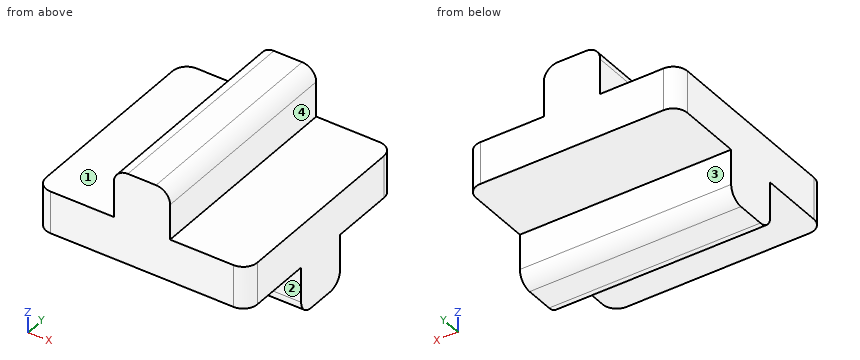
from build123d import *

# Parameters (mm, degrees)
SKETCH_1_W      = 30
SKETCH_1_H      = 30
EXTRUDE_1_DEPTH = 6
SKETCH_2_W      = 30
SKETCH_2_H      = 8
EXTRUDE_2_DEPTH = 7
FILLET_1_R      = 2
FILLET_2_R      = 2
SKETCH_3_W      = 8
SKETCH_3_H      = 30
EXTRUDE_3_DEPTH = 7
FILLET_3_R      = 2


with BuildPart() as part:
    # 스케치1 → 보스-돌출1 (new body)
    with BuildSketch(Plane.XY):
        Rectangle(SKETCH_1_W, SKETCH_1_H)
    extrude(amount=EXTRUDE_1_DEPTH)

    # 스케치2 → 보스-돌출2 (add)
    with BuildSketch(Plane(origin=(0, 0, 0), x_dir=(-1, 0, 0), z_dir=(0, 0, -1))):
        Rectangle(SKETCH_2_W, SKETCH_2_H)
    extrude(amount=EXTRUDE_2_DEPTH)

    # 필렛1
    fillet_1_edges = [part.edges().sort_by_distance(p)[0] for p in [
        (0, 4, -7),
        (0, -4, -7),
    ]]
    fillet(fillet_1_edges, radius=FILLET_1_R)

    # 필렛2
    fillet_2_edges = [part.edges().sort_by_distance(p)[0] for p in [
        (15, -15, 3),
        (-15, -15, 3),
        (-15, 15, 3),
        (15, 15, 3),
    ]]
    fillet(fillet_2_edges, radius=FILLET_2_R)

    # 스케치3 → 보스-돌출3 (add)
    with BuildSketch(Plane.XY.offset(6)):
        Rectangle(SKETCH_3_W, SKETCH_3_H)
    extrude(amount=EXTRUDE_3_DEPTH)

    # 필렛3
    fillet_3_edges = [part.edges().sort_by_distance(p)[0] for p in [
        (4, 0, 13),
        (-4, 0, 13),
    ]]
    fillet(fillet_3_edges, radius=FILLET_3_R)


solid = part.part
Can you work these out from the model? Positions are in its coordinate system, mm. Face numbers are marked on the shaded views. A direction names the side the tool comes from. Give positions to 0.01 mm unless a question says otherwise; leave off trailing zeros. Order: outer loops, then holes, each group sorted by start corner. A loop starts at its lowest first (then second) coordinate and runs counter-clockwise, first axis right, second up. Notation, with made-up numbers: M -13.75,89.5 L 9.25,89.5 A20 ccw 9.25,95.5 Z; hole C 57,33.25 d9. An arc over 180 degrees is marked long. Use a Markdown table: item, result. Add a question column.
Item 1: Suppose I cut it at C-C (z = 9). List the corners of the cut face in (x, y) for me, then the cut area to 3 significant figures.
Item 2: If I drill on L1, parallel to X at y = 12, z = 10; L2, parallel to Z at x = -6, y = -5; L3, parallel to Z at x = 0.25, y = -12.75, over which ranges is the centre line in solid material (lowest first)? Write a range as [from, to].
Item 3: Suppose I cut it at D-D (z = 11.5). List the corners of the cut face in (x, y) for me.
Item 4: For the marked faces 1, 2, 3 and 4, which set-ups out of +Z, -Z, +X, -X, +Y, -Y let a thin tool reach every point of the face, with its end or its side?
Item 5: Suppose I cut it at A-A (y = 5.75). List the corners of the cut face in (x, z) for me.
Item 6: Suppose I cut it at B-B (x = -7.75). List the corners of the cut face in (y, z) for me.
Item 7: Will these pins go through, and if not, where does the flat tip stop? pin 1 (3.5 mm diameter, centred on x = 7.5, y = -3, fed in from +Z); pin 2 (12 mm diameter, centred on x = -1.5, y = 11.5, fed in from -Z); pin 3 (1.5 mm diameter, centred on y = -6.5, z = 7.5, fed in from +X).
Answer sheet:
| question | item | result |
|---|---|---|
| 1 | outline | M -4,-15 L 4,-15 L 4,15 L -4,15 Z |
| 1 | area | 240 mm² |
| 2 | L1 | x = [-4, 4] |
| 2 | L2 | z = [0, 6] |
| 2 | L3 | z = [0, 13] |
| 3 | outline | M -3.94,-15 L 3.94,-15 L 3.94,15 L -3.94,15 Z |
| 4 | face 1 | +Z, -X, +Y, -Y |
| 4 | face 2 | -Z, +X, -X, -Y |
| 4 | face 3 | -Z, +X, -X, +Y |
| 4 | face 4 | +Z, +X, +Y, -Y |
| 5 | outline | M -15,0 L 15,0 L 15,6 L 4,6 L 4,11 A2 ccw 2,13 L -2,13 A2 ccw -4,11 L -4,6 L -15,6 Z |
| 6 | outline | M -15,0 L -4,0 L -4,-5 A2 ccw -2,-7 L 2,-7 A2 ccw 4,-5 L 4,0 L 15,0 L 15,6 L -15,6 Z |
| 7 | pin 1 | stops at z = 6 |
| 7 | pin 2 | stops at z = 0 |
| 7 | pin 3 | stops at x = 4 |
